Input: part model. Units: mm. Frame: model coordinates. A direction names the side the tool comes from. Coordinates: 2 decimals unless noted, no trailing zeros. Write each loop counter-clockwise with the first axis right and the second up, starting at its lowest first coordinate (ties: lowest second). Pieces come first, ordered by that corner, then holes. Notation, with made-up numbers: (-29.75, 12.25) - (-2.75, 12.25) arc R35 cw to (-2.75, 47.25) - close; hole circle Ø6 at (52.25, 84). An arc over 180 degrees is marked (long way). Use a Markdown table: item, result. Add a question column.
Q1. Material intervals for probe 1 along Z at (x, y) = (714.5, 6.25), sorted ascending. Write a range as from..to.
Q2. Set-up query: faces 1 (the face through (618, 0, -493)), 2 (the face through (523.714, 0.493, -450.7)). Return all of +Z, -Z, +X, -X, +Y, -Y with unobstructed straight access to the full face (end or side cutting, diameter ignored); none if empty.
Q3. Mould query, pull axis Z, two halves, no side actions, for faces 3 (the face through (507, 17, -493)), 4 (the face through (623.364, 0.493, -549.3)). Classes: released by +Z, released by -Z, zero draft, split by the parting line, or undercut.
Q4. Section query B-B (x = 301.5). Return the cut outline in (y, z).
Q5. Section query C-C (x = 869.5). Return the cut outline in (y, z).
Q6. Pin query (flat end, axial travel): P1, Ø5, axis at x = 836.5, y = 5, coming from the +Z side; P2, Ø0.8, axis at x = 581, y = 0.5, coming from the -Z side. Return the tip coordinate at first contact, or that it passes through.
Q7. Section query A-A (y = 8.5). Return the cut outline in (x, z).
Autodesk Inventor part; units mm, degrees
ref_plane "YZ Plane" through (0, 0, 0) normal (1, 0, 0) x (0, 1, 0)
ref_plane "XZ Plane" through (0, 0, 0) normal (0, 1, 0) x (-1, 0, 0)
ref_plane "XY Plane" through (0, 0, 0) normal (0, 0, 1) x (1, 0, 0)
sketch "Boceto1" plane through (0, 0, 0) normal (0, 1, 0) x (-1, 0, 0)
  line L0 (0, 0) -> (-1000, 0)
  line L1 (-1000, 0) -> (-1000, -1000)
  line L2 (-1000, -1000) -> (0, -1000)
  line L3 (0, -1000) -> (0, 0)
  dimension "d0" = 1000
  dimension "d1" = 1000
extrude "Extrusión1" add sketch "Boceto1" along normal blind 17
sketch "Boceto2" plane through (0, 0, 0) normal (0, -1, 0) x (1, 0, 0)
  line L0 (286.7389, -300) -> (686.7389, -300)
  line L1 (0, 0) -> (1000, 0)
  line L2 (686.7389, -700) -> (286.7389, -700)
  line L3 (1000, -1000) -> (0, -1000)
  line L4 (686.7389, -300) -> (686.7389, -400)
  line L5 (286.7389, -300) -> (286.7389, -300)
  line L6 (286.7389, -300) -> (286.7389, -400)
  line L7 (286.7389, -700) -> (286.7389, -600)
  line L8 (686.7389, -700) -> (686.7389, -600)
  line L9 (286.7389, -400) -> (561.7389, -400)
  line L10 (286.7389, -600) -> (561.7389, -600)
  line L11 (561.7389, -600) -> (486.7389, -500)
  line L12 (486.7389, -500) -> (561.7389, -400)
  line L13 (686.7389, -400) -> (561.7389, -500)
  line L14 (561.7389, -500) -> (686.7389, -600)
  dimension "d4" = 300
  dimension "d5" = 300
  dimension "d6" = 100
  dimension "d7" = 100
  dimension "d8" = 100
  dimension "d9" = 100
  dimension "d10" = 200
  dimension "d11" = 400
  dimension "d12" = 400
  dimension "d13" = 275
extrude "Extrusión2" cut sketch "Boceto2" against normal blind 1
sketch "Boceto3" plane through (0, 0, 0) normal (0, 0, 1) x (1, 0, 0)
  circle A0 centre (30, 8.5) radius 8.5
  line L0 (0, 0) -> (1000, 0)
  circle A1 centre (970, 8.5) radius 8.5
  line L1 (0, 0) -> (0, 17)
  line L2 (1000, 0) -> (1000, 17)
  dimension "d17" = 17
  dimension "d18" = 17
  dimension "d21" = 30
  dimension "d22" = 30
extrude "Extrusión3" add sketch "Boceto3" along normal blind 50
sketch "Boceto5" plane through (1000, 0, -1000) normal (0, 0, -1) x (-1, 0, 0)
  circle A0 centre (30, 8.5) radius 8.5
  circle A1 centre (30, 8.5) radius 8.5
  line L0 (0, 0) -> (0, 17)
  arc A2 (970, 0) -> (970, 17) centre (970, 8.5) ccw
  circle A3 centre (970, 8.5) radius 8.5
  line L1 (1000, 0) -> (1000, 17)
  line L2 (0, 0) -> (1000, 0)
  dimension "d23" = 30
  dimension "d24" = 30
extrude "Extrusión4" add sketch "Boceto5" along normal blind 50
properties part number "01_10_Plataforma" material "Acero ASTM A36"
Values follow:
| question | item | result |
|---|---|---|
| 1 | probe 1 | -1000..0 |
| 2 | face 1 | +Z, -Z, +X, -X, -Y |
| 2 | face 2 | -Y |
| 3 | face 3 | zero draft |
| 3 | face 4 | undercut |
| 4 | outline | (0, -1000) - (17, -1000) - (17, 0) - (0, 0) - (0, -300) - (1, -300) - (1, -400) - (0, -400) - (0, -600) - (1, -600) - (1, -700) - (0, -700) - close |
| 5 | outline | (0, -1000) - (17, -1000) - (17, 0) - (0, 0) - close |
| 6 | P1 | z = 0 |
| 6 | P2 | z = -1000 |
| 7 | outline | (0, -1000) - (21.5, -1000) - (21.5, -1050) - (38.5, -1050) - (38.5, -1000) - (961.5, -1000) - (961.5, -1050) - (978.5, -1050) - (978.5, -1000) - (1000, -1000) - (1000, 0) - (978.5, 0) - (978.5, 50) - (961.5, 50) - (961.5, 0) - (38.5, 0) - (38.5, 50) - (21.5, 50) - (21.5, 0) - (0, 0) - close |
